Work out the finished part from the listing and answer in its coordinate system (mm). A direction names the side the tool comes from. Round coordinates to 2 decimals unless told otherwise and drop trailing zeros. Order: outer loops, then holes, each group sorted by start corner. A loop starts at its lowest first (then second) coordinate and runs counter-clockwise, first axis right, second up. Notation, with made-up numbers: (69.25, 80.5) - (128.25, 80.5) arc R38 cw to (128.25, 118.5) - close; hole circle Ø1 at (-9.75, -38.5). An arc over 180 degrees is marked (long way). Put each result on its own line as item: value.
Autodesk Inventor part; units mm, degrees
ref_plane "YZ Plane" through (0, 0, 0) normal (1, 0, 0) x (0, 1, 0)
ref_plane "XZ Plane" through (0, 0, 0) normal (0, 1, 0) x (-1, 0, 0)
ref_plane "XY Plane" through (0, 0, 0) normal (0, 0, 1) x (1, 0, 0)
ref_plane "Work Plane1" through (0, 0, 0) normal (0, 0, 1) x (1, 0, 0)
sketch "Sketch1" plane through (0, 0, 0) normal (0, 0, 1) x (1, 0, 0)
  line L0 (21.9816, 24.6798) -> (-20.9074, 24.6798)
  line L1 (-20.9074, 24.6798) -> (-20.9074, -5.2231)
  line L2 (-20.9074, -5.2231) -> (21.9816, -5.2231)
  line L3 (21.9816, -5.2231) -> (21.9816, 24.6798)
  line L4 (-10.9398, 24.6798) -> (-10.9398, -5.2231)
  line L5 (11.8882, 24.6798) -> (11.8882, -5.2231)
  circle A0 centre (19.7466, 22.1825) radius 1.5378
  circle A1 centre (19.7466, -3.0178) radius 1.5307
  circle A2 centre (-18.5031, -1.487) radius 1.5327
  circle A3 centre (-18.5031, 22.1825) radius 1.5785
  point P0 (0, 0)
ref_plane "Work Plane2" through (0, 0, 0) normal (0, 0, 1) x (1, 0, 0)
extrude "Extrusion1" add sketch "Sketch1" along normal blind 3.65 contours L3 L2 L5 L0 | L4 L2 L1 L0
sketch "Sketch3" plane through (0, 0, 3.65) normal (0, 0, 1) x (1, 0, 0)
  line L0 (11.8882, 24.6798) -> (11.8882, -5.2231)
  line L1 (21.9816, 24.6798) -> (11.8882, 24.6798)
  line L2 (11.8882, -5.2231) -> (15.3769, -5.2231)
  line L3 (15.3769, -5.2231) -> (15.3769, 24.6798)
  line L4 (15.3769, 24.6798) -> (11.8882, 24.6798)
  line L5 (11.8882, 24.6798) -> (11.8882, -5.2231)
  line L6 (-10.9398, 24.6798) -> (-20.9074, 24.6798)
  line L7 (-10.9398, -5.2231) -> (-13.9699, -5.2231)
  line L8 (-13.9699, -5.2231) -> (-13.9699, 24.6798)
  line L9 (-13.9699, 24.6798) -> (-10.9398, 24.6798)
  line L10 (-10.9398, 24.6798) -> (-10.9398, -5.2231)
  point P0 (0, 0)
extrude "Extrusion2" add sketch "Sketch3" along normal blind 19.525
sketch "Sketch4" plane through (-10.9398, -5.2231, 0) normal (1, 0, 0) x (0, 0, -1)
  line L0 (0, 0) -> (-23.175, 0)
  line L1 (0, 29.9028) -> (-23.175, 29.9028)
  line L2 (-23.175, 0) -> (-19.0955, 0)
  line L3 (-19.0955, 0) -> (-19.0955, 29.9028)
  line L4 (-19.0955, 29.9028) -> (-23.175, 29.9028)
  line L5 (-23.175, 29.9028) -> (-23.175, 0)
  point P0 (0, 5.2231)
extrude "Extrusion3" add sketch "Sketch4" along normal up to surface (22.828 mm away)
properties part number "MotorLock"
1) Given pin 1 Ø5 at (x, y) = (19.75, 22.18) entering from +Z; pin 2 Ø7 at (y, z) = (16, 14) entering from -X; pin 3 Ø3 at (y, z) = (8.5, 9.5) entering from +X, each flat-ended and moving along its own axis, determine where each tip first touches the part or whether it passes through.
Findings below:
pin 1: stops at z = 3.65
pin 2: stops at x = -13.97
pin 3: stops at x = 15.38
2) Straight lines are drawn through the part: L1, parallel to X at y = 0.75, z = 1; L2, parallel to X at y = 20.5, z = 4.75; L3, parallel to Z at x = -2.5, y = 12 (1 decimal). For each, find the intervals that lie inside material, in ascending order. Write a range as from..to.
Findings below:
L1: x = -20.91..-10.94, 11.89..21.98
L2: x = -13.97..-10.94, 11.89..15.38
L3: z = 19.1..23.2
3) A cutting plane is placed at B-B on y = 21.25. Give the number of separate pieces and of enclosed holes in the cut face, then the cut area to 3 significant figures.
Findings below:
separate pieces: 3
enclosed holes: 0
area: 275 mm2
4) A cutting plane is placed at A-A on z = 14.25. Write down the section's boundary in (x, y), then the cut area to 3 significant figures.
Findings below:
outline: (-13.97, -5.22) - (-10.94, -5.22) - (-10.94, 24.68) - (-13.97, 24.68) - close; (11.89, -5.22) - (15.38, -5.22) - (15.38, 24.68) - (11.89, 24.68) - close
area: 195 mm2
5) For faces 5 (the flat face through (15.377, 10, 13)), 6 (the flat face through (-10.94, 10, 9)), 7 (the cylindrical face through (21.16, -2.43, 1.8)), 8 (the flat face through (-17, 10, 3.65)), determine the directions among +Z, -Z, +X, -X, +Y, -Y from which every point of the face is accessible in a straight line to the end or side of a thin tool.
Findings below:
face 5: +Z, +X, +Y, -Y
face 6: -Z, +Y, -Y
face 7: +Z, -Z
face 8: +Z, -X, +Y, -Y
6) For a pull along Y with two mould halves and no side action, classify faces 1 (the cylindrical face through (-17.655, 20.852, 1.799)), 2 (the flat face through (17, 10, 0)), 3 (the flat face through (-13.6, 24.68, 8.9)), 4 (the flat face through (3.6, -5.223, 19.3)) as pulls with the +Y half, pulls with the -Y half, needs draft (parallel to the pull), parting line crosses it, or undercut.
Findings below:
face 1: undercut
face 2: needs draft
face 3: pulls with the +Y half
face 4: pulls with the -Y half
